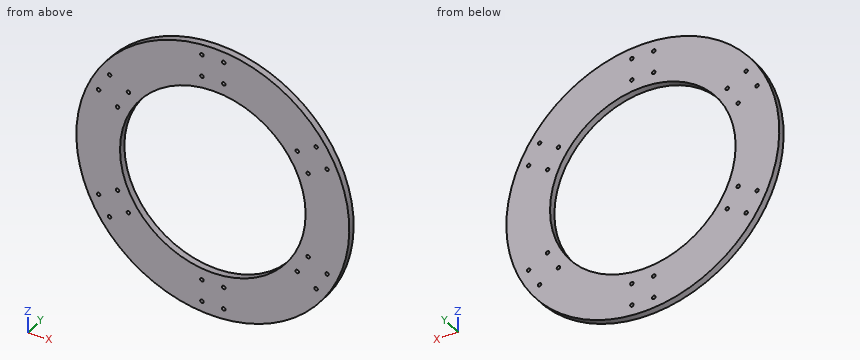
```python
from build123d import *

# Parameters (mm, degrees)
SKETCH1_R            = 125
BOSS_EXTRUDE1_DEPTH  = 6.35
SKETCH2_R            = 85
CUT_EXTRUDE1_DEPTH   = 177.890707783
M3_CLEARANCE_HOLE1_D = 3.2


with BuildPart() as part:
    # Sketch1 → Boss-Extrude1 (new body)
    with BuildSketch(Plane(origin=(0, 0, 0), x_dir=(1, 0, 0), z_dir=(0, 1, 0))):
        with Locations(Location((0, 0, 0), (0, 0, 270))):
            Circle(SKETCH1_R)
    extrude(amount=BOSS_EXTRUDE1_DEPTH)

    # Sketch2 → Cut-Extrude1 (cut, through all)
    with BuildSketch(Plane(origin=(0, 0, 0), x_dir=(1, 0, 0), z_dir=(0, 1, 0))):
        with Locations(Location((0, 0, 0), (0, 0, 270))):
            Circle(SKETCH2_R)
    extrude(amount=CUT_EXTRUDE1_DEPTH, mode=Mode.SUBTRACT)

    # M3 Clearance Hole1 (through all)
    with Locations(Plane(origin=(0, 0, 0), x_dir=(-1, 0, 0), z_dir=(0, -1, 0))):
        with Locations((10, -95), (-10, -95), (10, -115), (-10, -115), (-77.27241336, -56.160254038), (-87.27241336, -38.839745962), (-94.592921435, -66.160254038), (-104.592921435, -48.839745962), (-87.27241336, 38.839745962), (-77.27241336, 56.160254038), (-104.592921435, 48.839745962), (-94.592921435, 66.160254038), (0, 0), (-10, 95), (10, 95), (-10, 115), (10, 115), (77.27241336, 56.160254038), (87.27241336, 38.839745962), (94.592921435, 66.160254038), (104.592921435, 48.839745962), (87.27241336, -38.839745962), (77.27241336, -56.160254038), (104.592921435, -48.839745962), (94.592921435, -66.160254038)):
            Hole(M3_CLEARANCE_HOLE1_D / 2)


solid = part.part
```
The listing builds one solid part. Answer for the finished solid, in the listing's coordinates (mm). Give positions to 0.01 mm unless a question says otherwise; leave off trailing zeros. Write each loop counter-clockwise with the first axis right and the second up, starting at its lowest first coordinate (ties: lowest second). Pieces come first, ordered by that corner, then holes. Notation, with made-up numbers: (-13.5, 62.25) - (-2.5, 62.25) arc R29 ccw to (-2.5, 86.25) - close; hole circle Ø7 at (26.5, 60). An arc over 180 degrees is marked (long way). Use one line per item in the form item = value. Start each with the question number.
1) Consider line 1 along X through (y, z) = (3, 115); line 2 along Z through (x, y) = (-10, 2.5); line 3 along X through (y, z) = (1.25, -39). Determine where each line is inside the solid, lowest interval first. Write a range as from..to.
2) Find section B-B on z = -8.5. Determine the outline of the cut face in (x, y), plus the area to 3 significant figures.
3) Find section D-D on z = 88.5. Determine the outline of the cut face in (x, y), plus the area to 3 significant figures.
4) Find section C-C on y = 1. Count the separate pieces of the cut face and the enclosed holes in it, plus the area to 3 significant figures.
5) Flat-ended cylindrical pins translate along their axes: pin 1 Ø1 at (y, z) = (4, -59) entering from -X; pin 2 Ø3 at (x, y) = (19.5, 5.5) entering from +Z; pin 3 Ø3 at (x, y) = (-65.5, 1.5) entering from -Z. Find the tip coordinate at first contact, or state that the pin passes through.
6) Find section A-A on x = 0. Determine the outline of the cut face in (y, z), plus the area to 3 significant figures.
Geometry results:
q1.line_1 = -48.99..-11.6, -8.4..8.4, 11.6..48.99
q1.line_2 = -124.6..-116.6, -113.4..-96.6, -93.4..-84.41, 84.41..93.4, 96.6..113.4, 116.6..124.6
q1.line_3 = -118.76..-88.86, -85.68..-75.52, 75.52..85.68, 88.86..118.76
q2.outline = (-124.71, 0) - (-84.57, 0) - (-84.57, 6.35) - (-124.71, 6.35) - close; (84.57, 0) - (124.71, 0) - (124.71, 6.35) - (84.57, 6.35) - close
q2.area = 510 mm2
q3.outline = (-88.28, 0) - (88.28, 0) - (88.28, 6.35) - (-88.28, 6.35) - close
q3.area = 1,120 mm2
q4.separate_pieces = 1
q4.enclosed_holes = 25
q4.area = 26,200 mm2
q5.pin_1 = -110.47
q5.pin_2 = 123.7
q5.pin_3 = -107.37
q6.outline = (0, -125) - (6.35, -125) - (6.35, -85) - (0, -85) - close; (0, 85) - (6.35, 85) - (6.35, 125) - (0, 125) - close
q6.area = 508 mm2
